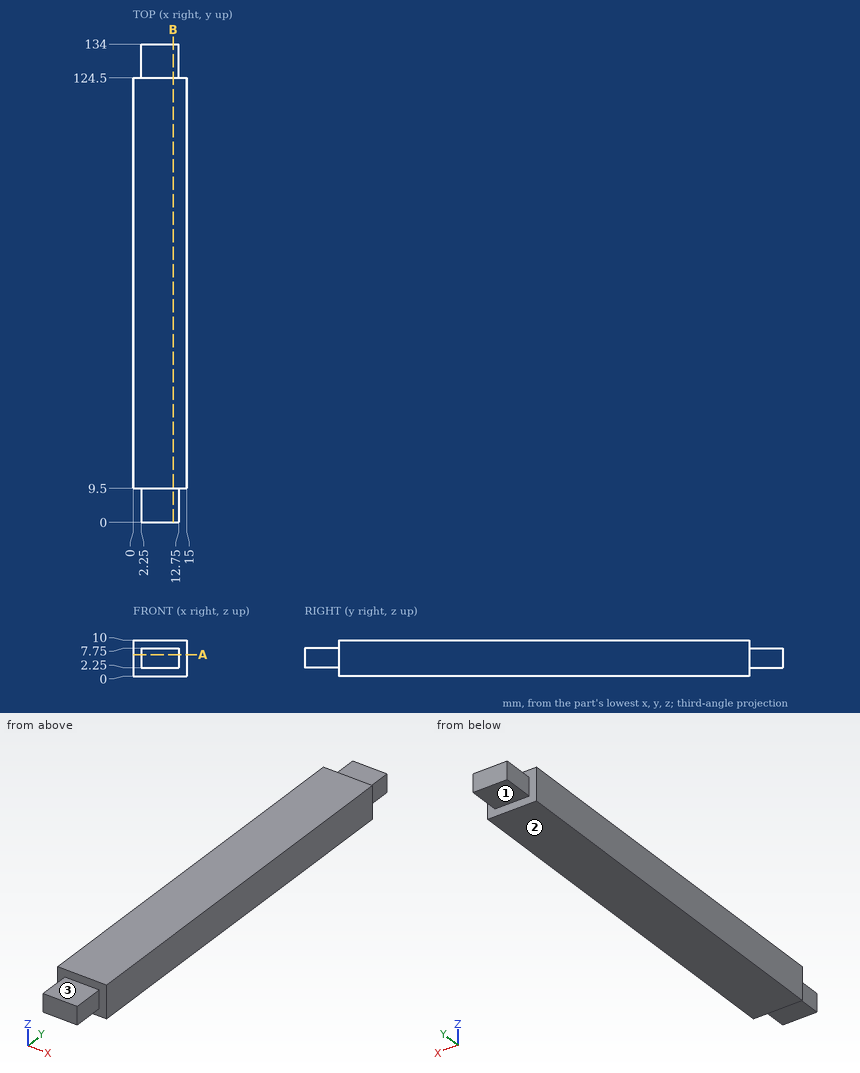
Drawing for the job (mm, zero at the part's lowest x, y, z). A direction names the side the tool comes from. Round coordinates to 2 decimals unless told otherwise and drop trailing zeros. Write each loop counter-clockwise with the first axis right and the second up, starting at its lowest first coordinate (ties: lowest second). Pieces come first, ordered by that corner, then holes. Notation, with made-up numbers: M 9.25,87.25 L 63.25,87.25 A17 cw 63.25,118.25 Z; hole C 43.25,52.5 d8. An arc over 180 degrees is marked long. One line per question, with ' | ' between items.
1. Cut at A-A on z = 6. Write the cut outline in (x, y), and give its area (3 significant figures).
Working result:
outline: M 0,9.5 L 2.25,9.5 L 2.25,0 L 12.75,0 L 12.75,9.5 L 15,9.5 L 15,124.5 L 12.75,124.5 L 12.75,134 L 2.25,134 L 2.25,124.5 L 0,124.5 Z | area: 1,920 mm2
2. Which spindle directions (+Z, -Z, +X, -X, +Y, -Y) get a long thin tool onto all of the face, cutting with end or side? Do the marked faces 1, 2 and 3. Say none if no direction does.
Working result:
face 1: -Z, +X, -X, +Y | face 2: -Z, +X, -X, +Y, -Y | face 3: +Z, +X, -X, -Y
3. Cut at B-B on x = 11.25. Write the cut outline in (y, z), and give its area (3 significant figures).
Working result:
outline: M 0,2.25 L 9.5,2.25 L 9.5,0 L 124.5,0 L 124.5,2.25 L 134,2.25 L 134,7.75 L 124.5,7.75 L 124.5,10 L 9.5,10 L 9.5,7.75 L 0,7.75 Z | area: 1,250 mm2
4. Pin check, flat tips, straight feed: pin 1 Ø1.6 at (y, z) = (5, 4) entering from +X; pin 2 Ø3 at (x, z) = (5, 5) entering from -Y; pin 3 Ø5 at (x, y) = (8.5, 130.5) entering from -Z; pin 4 Ø4.5 at (y, z) = (130, 4) entering from -X. Stop position of each tip, or through.
Working result:
pin 1: x = 12.75 | pin 2: y = 0 | pin 3: z = 2.25 | pin 4: x = 2.25
5. Probe L1, parallel to Y at x = 11, z = 9.75; L2, parallel to X at y = 7.5, z = 4.25; L3, parallel to Z at x = 4.5, y = 7. List the from-to ranges inside material, lowest first. Write a range as from..to.
Working result:
L1: 9.5..124.5 | L2: 2.25..12.75 | L3: 2.25..7.75
